Can you work these out from the model? Positions are in its coordinate system, mm. Give positions to 0.01 mm unless a question says otherwise; leave off trailing zeros. Write each loop counter-clockwise with the first axis right and the second up, starting at its lowest first coordinate (ties: lowest second). Pieces come first, ordered by that corner, then holes.
```python
from build123d import *

# Parameters (mm, degrees)
EXTRUDE_1_DEPTH       = 3
HOLE_WIZARD_3_0_3_1_D = 3
SKETCH_7_W            = 90
SKETCH_7_H            = 25
CUT_EXTRUDE_1_DEPTH   = 128.314571044
FILLET_7_R            = 10
HOLE_WIZARD_3_0_3_2_D = 3
SKETCH1_W             = 10
SKETCH1_H             = 40
CUT_EXTRUDE1_DEPTH    = 128.314571044
FILLET1_R             = 3


with BuildPart() as part:
    # Эскиз1 → Бобышка-Вытянуть1 (new body)
    with BuildSketch(Plane.XY):
        with BuildLine():
            Line((75, -90), (-75, -90))
            ThreePointArc((-75, -90), (-85.606601718, -85.606601718), (-90, -75))
            Line((-90, -75), (-90, 75))
            ThreePointArc((-90, 75), (-85.606601718, 85.606601718), (-75, 90))
            Line((-75, 90), (75, 90))
            ThreePointArc((75, 90), (85.606601718, 85.606601718), (90, 75))
            Line((90, 75), (90, -75))
            ThreePointArc((90, -75), (85.606601718, -85.606601718), (75, -90))
        make_face()
    extrude(amount=EXTRUDE_1_DEPTH)

    # Диаметр отверстия Ø3.0 (3)1 (through all)
    with Locations(Plane.XY.offset(3)):
        with Locations((-10, -24.15), (40.8, 8.85), (40.8, -19.05), (-8.5, 24.05)):
            Hole(HOLE_WIZARD_3_0_3_1_D / 2)

    # Эскиз7 → Вырез-Вытянуть1 (cut, through all)
    with BuildSketch(Plane.XY.offset(3)):
        with Locations((0, 77.5)):
            Rectangle(SKETCH_7_W, SKETCH_7_H)
        with Locations((0, -77.5)):
            Rectangle(SKETCH_7_W, SKETCH_7_H)
    extrude(amount=-CUT_EXTRUDE_1_DEPTH, mode=Mode.SUBTRACT)

    # Скругление7
    fillet_7_edges = [part.edges().sort_by_distance(p)[0] for p in [
        (-45, 65, 1.5),
        (-45, 90, 1.5),
        (45, 90, 1.5),
        (45, 65, 1.5),
        (-45, -90, 1.5),
        (-45, -65, 1.5),
        (45, -65, 1.5),
        (45, -90, 1.5),
    ]]
    fillet(fillet_7_edges, radius=FILLET_7_R)

    # Диаметр отверстия Ø3.0 (3)2 (through all)
    with Locations(Plane.XY.offset(3)):
        with Locations((-65, -65), (65, -65), (65, 65), (-65, 65)):
            Hole(HOLE_WIZARD_3_0_3_2_D / 2)

    # Sketch1 → Cut-Extrude1 (cut, through all)
    with BuildSketch(Plane.XY.offset(3)):
        with Locations((-40, 0)):
            Rectangle(SKETCH1_W, SKETCH1_H)
    extrude(amount=-CUT_EXTRUDE1_DEPTH, mode=Mode.SUBTRACT)

    # Fillet1
    fillet1_edges = [part.edges().sort_by_distance(p)[0] for p in [
        (-35, 20, 1.5),
        (-35, -20, 1.5),
        (-45, -20, 1.5),
        (-45, 20, 1.5),
    ]]
    fillet(fillet1_edges, radius=FILLET1_R)


solid = part.part
```
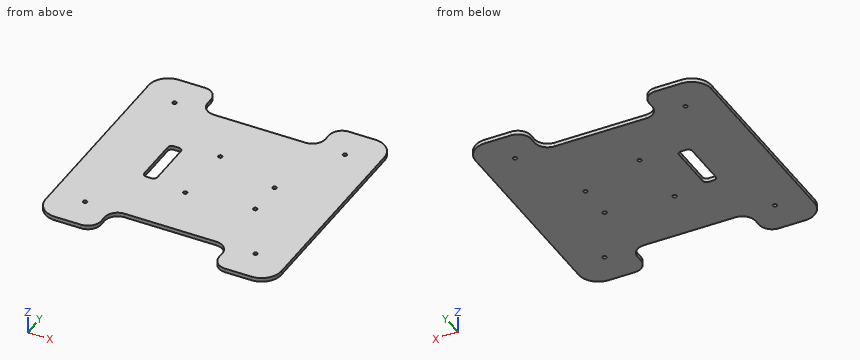
1) Suppose I cut it at A-A on z = 2.3. State how many separate pieces and enclosed holes the cut face has, plus the area to 3 significant figures.
Values follow:
separate pieces: 1
enclosed holes: 9
area: 27,300 mm2
2) For pin 1 Ø1.5 at (x, z) = (-40.5, 1) entering from +Y; pin 2 Ø1.5 at (x, z) = (-28.5, 0.5) entering from -Y; pin 3 Ø0.9 at (y, z) = (-78.5, 1) entering from +X, each with a flat end and sliding along its axis, tell me the tip position at first contact or that it passes through.
Values follow:
pin 1: stops at y = 67.19
pin 2: stops at y = -65
pin 3: stops at x = 89.69
3) Suppose I cut it at B-B on x = -27.5. Write out the boundary of the cut face in (y, z), plus the area to 3 significant figures.
Values follow:
outline: (-65, 0) - (65, 0) - (65, 3) - (-65, 3) - close
area: 390 mm2
4) Please list where these lines run through material, in increasing order: L1, parallel to Y at x = 64.5, z = 0.8; L2, parallel to Y at x = -26, z = 0.2; L3, parallel to X at y = 14.5, z = 1.95.
Values follow:
L1: y = -90 to -66.41, -63.59 to 63.59, 66.41 to 90
L2: y = -65 to 65
L3: x = -90 to -45, -35 to 90
